```python
from build123d import *

# Parameters (mm, degrees)
F1_DEPTH = 2590
F2_R     = 8
F3_DEPTH = 25


with BuildPart() as f1:
    # F0 (on Front) → F1 (new body)
    with BuildSketch(Plane.XZ):
        with BuildLine():
            Line((-35, -20), (35, -20))
            ThreePointArc((35, -20), (42.071068, -17.071068), (45, -10))
            Line((45, -10), (42.904106, -2.792146))
            ThreePointArc((42.904106, -2.792146), (42.506393, 0), (42.904106, 2.792146))
            Line((42.904106, 2.792146), (45, 10))
            ThreePointArc((45, 10), (42.071068, 17.071068), (35, 20))
            Line((35, 20), (-35, 20))
            ThreePointArc((-35, 20), (-42.071068, 17.071068), (-45, 10))
            Line((-45, 10), (-42.904106, 2.792146))
            ThreePointArc((-42.904106, 2.792146), (-42.506393, 0), (-42.904106, -2.792146))
            Line((-42.904106, -2.792146), (-45, -10))
            ThreePointArc((-45, -10), (-42.071068, -17.071068), (-35, -20))
        make_face()
    extrude(amount=F1_DEPTH)

    # F2 (on face) → F3 (cut)
    with BuildSketch(Plane(origin=(0, 0, -20), x_dir=(1, 0, 0), z_dir=(0, 0, -1))):
        with Locations((0, 2552.515268)):
            Circle(F2_R)
    extrude(amount=-F3_DEPTH, mode=Mode.SUBTRACT)


solid = f1.part
```
The listing builds one solid part. Answer for the finished solid, in the listing's coordinates (mm). Give positions to 0.01 mm unless a question says otherwise; leave off trailing zeros. Order: outer loops, then holes, each group sorted by start corner. A loop starts at its lowest first (then second) coordinate and runs counter-clockwise, first axis right, second up. Notation, with made-up numbers: (17.5, -9) -> (52.5, -9) arc R16 cw to (52.5, 7) -> close; hole circle Ø5 at (-15.5, 85.5). An arc over 180 degrees is marked (long way). Write each question's results on one line, items separated by ' | '.
Q1. The part is cut by section A-A, the plane y = -1655. Give the vertices of the cut face in (x, z), and give its area (3 significant figures).
Checked values:
outline: (-45, -10) arc R10 ccw to (-35, -20) -> (35, -20) arc R10 ccw to (45, -10) -> (42.9, -2.79) arc R10 cw to (42.9, 2.79) -> (45, 10) arc R10 ccw to (35, 20) -> (-35, 20) arc R10 ccw to (-45, 10) -> (-42.9, 2.79) arc R10 cw to (-42.9, -2.79) -> close | area: 3,460 mm^2
Q2. Each of these flat-tipped pins is pushed along its axis until it touches: P1, Ø5, axis at y = -1319, z = 16, coming from the -X side; P2, Ø1.5, axis at x = 14.5, z = 7, coming from the +Y side; P3, Ø8, axis at x = 2.5, y = -2554, coming from the -Z side; P4, Ø8, axis at y = -660, z = 5, coming from the -X side. Where does it stop, or does it pass through?
Checked values:
P1: stops at x = -44.37 | P2: stops at y = 0 | P3: stops at z = 5 | P4: stops at x = -44.71
Q3. Straight lines are drawn through the part: probe 1 along Y at (x, z) = (0, -5.25); probe 2 along X at (y, z) = (-644.5, 2); probe 3 along Z at (x, y) = (-37.5, -1151). For each, find the intervals that lie inside material, in ascending order. Write a range as from..to.
Checked values:
probe 1: y = -2590..-2560.52, -2544.52..0 | probe 2: x = -42.71..42.71 | probe 3: z = -19.68..19.68
